from build123d import *

# Parameters (mm, degrees)
SKETCH_1_R          = 20
EXTRUDE_1_DEPTH     = 266.5
EXTRUDE_START       = 35
SKETCH_3_R          = 20
EXTRUDE_2_DEPTH     = 35
CUT_EXTRUDE_1_DEPTH = 25
SKETCH_5_R          = 5
CUT_EXTRUDE_2_DEPTH = 10


with BuildPart() as part:
    # 스케치1 → 보스-돌출1 (new body)
    with BuildSketch(Plane.XY):
        Circle(SKETCH_1_R)
    extrude(amount=EXTRUDE_1_DEPTH)

    # 스케치3 → 보스-돌출2 (add)
    with BuildSketch(Plane(origin=(0, 0, 0), x_dir=(-1, 0, 0), z_dir=(0, 0, -1)).offset(EXTRUDE_START)):
        Circle(SKETCH_3_R)
    extrude(amount=-EXTRUDE_2_DEPTH)

    # 스케치4 → 컷-돌출1 (cut)
    with BuildSketch(Plane(origin=(0, 0, -35), x_dir=(-1, 0, 0), z_dir=(0, 0, -1))):
        with BuildLine():
            Line((-3.515670801, 3.555286039), (-3.484261495, -3.586073317))
            ThreePointArc((-3.484261495, -3.586073317), (4.99995164, 0.021990913), (-3.515670801, 3.555286039))
        make_face()
    extrude(amount=-CUT_EXTRUDE_1_DEPTH, mode=Mode.SUBTRACT)

    # 스케치5 → 컷-돌출2 (cut)
    with BuildSketch(Plane(origin=(0, 0, -35), x_dir=(-1, 0, 0), z_dir=(0, 0, -1))):
        Circle(SKETCH_5_R)
    extrude(amount=-CUT_EXTRUDE_2_DEPTH, mode=Mode.SUBTRACT)


solid = part.part
Verification items for the finished model (mm, model axes). Round coordinates to 2 decimals unless told otherwise and drop trailing zeros. Loops run counter-clockwise (first coordinate to the right, second up) from the corner with the lowest first, then second, coordinate; pieces in that order, holes last. Notation, with made-up numbers: (18, 65) - (23, 65) arc R12 cw to (23, 86) - close; hole circle Ø7 at (7, -7). An arc over 180 degrees is marked (long way). Answer in a Markdown table with one row per item. Add a question column.
Q1. Material ranges on line 1 (Y direction, x = 0, z = -16); line 2 (X direction, y = 0, z = -20); line 3 (Y direction, x = -0.5, z = 80), recorded low to high.
Q2. Section check B-B on z = 131. Enter the section's corners in (x, y), plus the area to 3 significant figures.
Q3. Section check D-D on y = -13.5. Enter the section's corners in (x, z), plus the area to 3 significant figures.
Q4. Gauge pin test, flat ends, axial feed: pin 1 (0.8 mm diameter, centred on x = 4, y = -0.5, fed in from -Z); pin 2 (3 mm diameter, centred on y = 6, z = 78.5, fed in from +X); pin 3 (1 mm diameter, centred on y = 3, z = 209, fed in from +X). Record the tip position at first contact, or that the pin passes through.
Q5. Section check C-C on y = 15.5. Enter the section's corners in (x, z).
Q6. Release check for a two-part mould opening along Y. For faces 1 (the face through (0, 0, 266.5)), 2 (the face through (-1, 0, -10)) record: pulls with the +Y half, pulls with the -Y half, needs draft (parallel to the pull), parting line crosses it, or undercut.
Q7. Section check A-A on x = 0. Enter the section's corners in (y, z).
Found:
| question | item | result |
|---|---|---|
| 1 | line 1 | y = -20 to -5, 5 to 20 |
| 1 | line 2 | x = -20 to -5, 3.5 to 20 |
| 1 | line 3 | y = -19.99 to 19.99 |
| 2 | outline | circle Ø40 at (0, 0) |
| 2 | area | 1,260 mm² |
| 3 | outline | (-14.76, -35) - (14.76, -35) - (14.76, 266.5) - (-14.76, 266.5) - close |
| 3 | area | 8,900 mm² |
| 4 | pin 1 | stops at z = -25 |
| 4 | pin 2 | stops at x = 19.49 |
| 4 | pin 3 | stops at x = 19.84 |
| 5 | outline | (-12.64, -35) - (12.64, -35) - (12.64, 266.5) - (-12.64, 266.5) - close |
| 6 | face 1 | needs draft |
| 6 | face 2 | undercut |
| 7 | outline | (-20, -35) - (-5, -35) - (-5, -10) - (5, -10) - (5, -35) - (20, -35) - (20, 266.5) - (-20, 266.5) - close |
